The listing builds one solid part. Answer for the finished solid, in the listing's coordinates (mm). Face numbers are marked on the shaded views. Give positions to 0.01 mm unless a question says otherwise; leave off trailing zeros. Write each loop counter-clockwise with the first axis right and the second up, starting at its lowest first coordinate (ties: lowest second). Pieces come first, ordered by that corner, then holes. Notation, with made-up numbers: (8, 52) - (14, 52) arc R4 ccw to (14, 57) - close; hole circle Ø5 at (73.25, -1). An arc over 180 degrees is marked (long way). Return JSON: item names as keys, results as strings.
from build123d import *

# Parameters (mm, degrees)
F3_DEPTH = 25
F4_R     = 0.5
F7_R     = 0.49999


# Not quite as in the source:
# - a fillet or chamfer is up to 0.001 mm smaller than in the source, because OpenCascade refuses the exact size


with BuildPart() as f1:
    # F0 (on Front) → F1 (revolve)
    with BuildSketch(Plane.XZ):
        with BuildLine():
            Line((-14.5, 0), (0, 0))
            Line((0, 0), (0, 94))
            Line((0, 94), (-8, 94))
            Line((-8, 94), (-8, 92.8))
            Line((-8, 92.8), (-12, 92.8))
            ThreePointArc((-12, 92.8), (-15.1799323999, 80.479338508), (-16.25, 67.8))
            Line((-16.25, 67.8), (-16.05, 67.8))
            Line((-16.05, 67.8), (-16.05, 67.75))
            Line((-16.05, 67.75), (-16.25, 67.75))
            Line((-16.25, 67.75), (-16.25, 66.75))
            Line((-16.25, 66.75), (-16.05, 66.75))
            Line((-16.05, 66.75), (-16.05, 66.7))
            Line((-16.05, 66.7), (-16.25, 66.7))
            Line((-16.25, 66.7), (-16.25, 43.8))
            Line((-16.25, 43.8), (-14.05, 43.8))
            Line((-14.05, 43.8), (-14.05, 39.7))
            Line((-14.05, 39.7), (-16.25, 39.7))
            ThreePointArc((-16.25, 39.7), (-15.8122876797, 19.8307240947), (-14.5, 0))
        make_face()
    revolve(axis=Axis((0, 0, 47), (0, 0, 1)))

    # F2 (on face) → F3 (cut)
    with BuildSketch(Plane(origin=(0, 0, 43.8), x_dir=(1, 0, 0), z_dir=(0, 0, -1))):
        with BuildLine():
            Line((11.7154812108, 4.5), (15.6144964696, 4.5))
            ThreePointArc((15.6144964696, 4.5), (0, 16.25), (-15.6144964696, 4.5))
            Line((-15.6144964696, 4.5), (-11.7154812108, 4.5))
            ThreePointArc((-11.7154812108, 4.5), (0, 12.55), (11.7154812108, 4.5))
        make_face()
    extrude(amount=F3_DEPTH, mode=Mode.SUBTRACT)

    # F4
    f4_edges = [f1.edges().sort_by_distance(p)[0] for p in [
        (8, 0, 94),
    ]]
    fillet(f4_edges, radius=F4_R)

    # F5 (on Front) → F6 (revolve)
    with BuildSketch(Plane.XZ):
        Polygon((14.5, 0), (0, 0), (0, -20), (10.55, -20), (10.55, -19), (10.95, -19), (14, -3), (14.5, -3), align=None)
    revolve(axis=Axis((0, 0, -10), (0, 0, -1)))

    # F7 (radius 0.5 in the source; OpenCascade refuses exactly that, so slightly less here)
    f7_edges = [f1.edges().sort_by_distance(p)[0] for p in [
        (-14.5, 0, -3),
    ]]
    fillet(f7_edges, radius=F7_R)


solid = f1.part
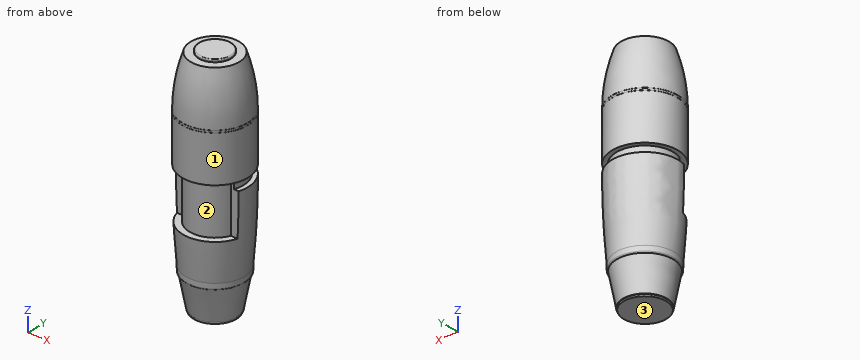
Item 1: A cutting plane is placed at A-A on z = 53. Determine the outline of the cut face in (x, y).
Answer below:
{"outline": "circle Ø32.5 at (0, 0)"}
Item 2: Flat-ended cylindrical pins translate along their axes: P1, Ø4, axis at y = -9.5, z = 73.5, coming from the -X side; P2, Ø2, axis at x = -11.5, y = -4, coming from the +Z side; P3, Ø1, axis at x = 9.5, z = 6.5, coming from the -Y side; P4, Ø8, axis at y = -3.5, z = 39.5, coming from the -X side. Find the tip coordinate at first contact, or state that the pin passes through.
Answer below:
{"P1": "stops at x = -14.19", "P2": "stops at z = 92.8", "P3": "stops at y = -12.04", "P4": "stops at x = -16.25"}
Item 3: Consider L1, parallel to Z at x = -2, y = 8.5; L2, parallel to X at y = 12.5, z = 1; L3, parallel to X at y = 0, z = 15.5. Determine where each line is inside the solid, lowest interval first.
Answer below:
{"L1": "z = -20 to 92.8", "L2": "x = -7.52 to 7.52", "L3": "x = -15.6 to 15.6"}
Item 4: The mould has two halves that part along Z. Classify the marked faces 1, 2 and 3: +Z half, -Z half, draft (parallel to the pull), parting line (faces both ways), or undercut.
Answer below:
{"face 1": "draft", "face 2": "undercut", "face 3": "-Z half"}
